Autodesk Inventor part; units mm, degrees
ref_plane "YZ Plane" through (0, 0, 0) normal (1, 0, 0) x (0, 1, 0)
ref_plane "XZ Plane" through (0, 0, 0) normal (0, 1, 0) x (-1, 0, 0)
ref_plane "XY Plane" through (0, 0, 0) normal (0, 0, 1) x (1, 0, 0)
sketch "Sketch1" plane through (0, 0, 0) normal (0, 1, 0) x (-1, 0, 0)
  line L0 (-35, 8) -> (-35, -8)
  line L1 (-35, -8) -> (35, -8)
  line L2 (35, -8) -> (35, 8)
  line L3 (35, 8) -> (-35, -8) construction
  line L4 (-35, 8) -> (35, -8) construction
  line L5 (-8, 8) -> (-8, 62)
  line L6 (-8, 62) -> (8, 62)
  line L7 (8, 62) -> (8, 8)
  line L8 (0, 0) -> (0, 99.8973) construction
  line L9 (35, 8) -> (8, 8)
  line L10 (-8, 8) -> (-35, 8)
  circle A0 centre (25, 3) radius 2.5
  circle A1 centre (10, -3) radius 2.5
  circle A2 centre (-10, -3) radius 2.5
  circle A3 centre (-25, 3) radius 2.5
  circle A4 centre (0, 22) radius 2.5
  circle A5 centre (0, 48) radius 2.5
  dimension "d0" = 70
  dimension "d1" = 16
  dimension "d2" = 16
  dimension "d4" = 70
  dimension "d5" = 5
  dimension "d6" = 5
  dimension "d7" = 5
  dimension "d8" = 10
  dimension "d10" = 10
  dimension "d11" = 10
  dimension "d12" = 10
  dimension "d13" = 14
  dimension "d14" = 40
extrude "Extrusion1" add sketch "Sketch1" along normal blind 1.2
equation "\"d10\" = d8"
equation "\"d11\" = d8"
equation "\"d12\" = d8"
equation "\"d13\" = 0.2 * d4"
equation "\"d14\" = 0.571429 * d4"
properties part number "FlatTee"
Verification items for the finished model (mm, model axes). Coordinates: 2 decimals unless noted, no trailing zeros. Order: outer loops, then holes, each group sorted by start corner. A loop starts at its lowest first (then second) coordinate and runs counter-clockwise, first axis right, second up. Notation, with made-up numbers: M -4.5,38 L 15.5,38 A22 cw 15.5,76 Z; hole C 52.5,-6 d11. An arc over 180 degrees is marked long. One line per item, written item: value. Start each with the question number.
Item 1: Depth check by flat-ended pin: P1, Ø0.6, axis at y = 1, z = 28, coming from the +X side. Enter the tip coordinate at first touch or a pass-through.
Item 2: Sectioned sample at D-D on z = 22. Record the cut outline in (x, y), then the cut area to 3 significant figures.
Item 3: Thickness scan on probe 1 along Z at (x, y) = (0, 0.85); probe 2 along Z at (x, y) = (-25, 0.7); probe 3 along X at (y, z) = (1.05, 15). Record the ranges inside material, lowest first.
Item 4: Sectioned sample at B-B on x = 25. Record the cut outline in (y, z).
Item 5: Sectioned sample at A-A on z = 4.5. Record the cut outline in (x, y), then the cut area to 3 significant figures.
Item 6: Sectioned sample at C-C on y = 1. Record the cut outline in (x, z).
Item 7: Mould release check, pull along X, two halves, no side actions. Record for faces 1 (the cylindrical face through (0.33, 0.59, 19.52)), 2 (the flat face through (0, 1.2, 19)): pulls with the +X half, pulls with the -X half, needs draft (parallel to the pull), parting line crosses it, or undercut.
Calculated:
1. P1: x = 8
2. outline: M -8,0 L -2.5,0 L -2.5,1.2 L -8,1.2 Z; M 2.5,0 L 8,0 L 8,1.2 L 2.5,1.2 Z
2. area: 13.2 mm^2
3. probe 1: -8 to 19.5, 24.5 to 45.5, 50.5 to 62
3. probe 2: -8 to 0.5, 5.5 to 8
3. probe 3: -8 to 8
4. outline: M 0,-8 L 1.2,-8 L 1.2,0.5 L 0,0.5 Z; M 0,5.5 L 1.2,5.5 L 1.2,8 L 0,8 Z
5. outline: M -35,0 L -27,0 L -27,1.2 L -35,1.2 Z; M -23,0 L 23,0 L 23,1.2 L -23,1.2 Z; M 27,0 L 35,0 L 35,1.2 L 27,1.2 Z
5. area: 74.4 mm^2
6. outline: M -35,-8 L 35,-8 L 35,8 L 8,8 L 8,62 L -8,62 L -8,8 L -35,8 Z; hole C -25,3 d5; hole C -10,-3 d5; hole C 0,22 d5; hole C 0,48 d5; hole C 10,-3 d5; hole C 25,3 d5
7. face 1: undercut
7. face 2: needs draft
